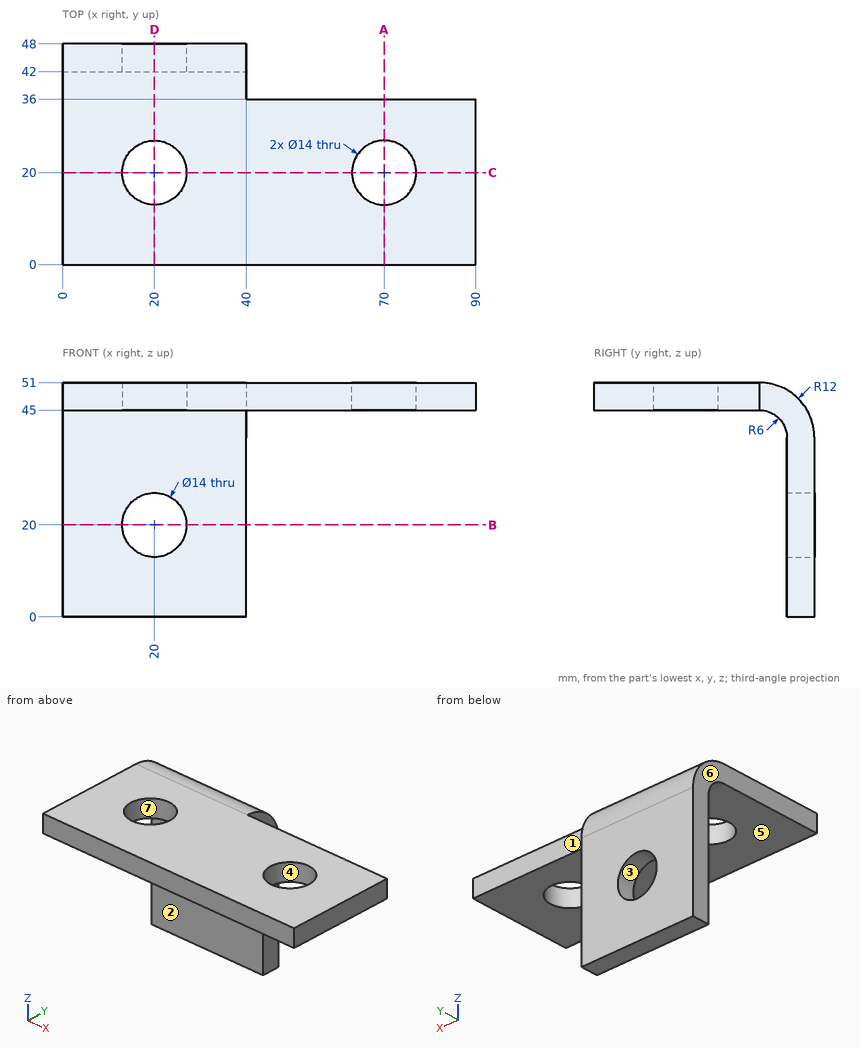
Drawing for the job (mm, zero at the part's lowest x, y, z). A direction names the side the tool comes from. Coordinates: 2 decimals unless noted, no trailing zeros. Order: outer loops, then holes, each group sorted by start corner. A loop starts at its lowest first (then second) coordinate and runs counter-clockwise, first axis right, second up. Notation, with made-up numbers: (-2.75, 26) -> (10.25, 26) arc R30 ccw to (10.25, 59) -> close; hole circle Ø5 at (51, 74.25). An arc over 180 degrees is marked (long way). Answer in a Markdown table with one row per item.
1) Drill centre lines: line 1 (X direction, y = 46.4, z = 20); line 2 (Y direction, x = 70, z = 47); line 3 (Z direction, x = 76.5, y = 23.5). Where is each one in solid material? Low to high.
Check values:
| item | result |
|---|---|
| line 1 | 0 to 13, 27 to 40 |
| line 2 | 0 to 13, 27 to 36 |
| line 3 | 45 to 51 |
2) Band-saw the part on C-C (y = 20). List the corners of the cut face in (x, z), and give its area (3 significant figures).
Check values:
| item | result |
|---|---|
| outline | (0, 45) -> (13, 45) -> (13, 51) -> (0, 51) -> close; (27, 45) -> (63, 45) -> (63, 51) -> (27, 51) -> close; (77, 45) -> (90, 45) -> (90, 51) -> (77, 51) -> close |
| area | 372 mm2 |
3) Band-saw the part on B-B (z = 20). List the corners of the cut face in (x, y), and give its area (3 significant figures).
Check values:
| item | result |
|---|---|
| outline | (0, 42) -> (13, 42) -> (13, 48) -> (0, 48) -> close; (27, 42) -> (40, 42) -> (40, 48) -> (27, 48) -> close |
| area | 156 mm2 |
4) Flat gauge pins, fed straight in: P1, Ø1.5, axis at x = 79.5, y = 24.5, coming from the -Z side; P2, Ø22.5, axis at x = 70, y = 20, coming from the +Z side; P3, Ø9.5, axis at y = 41.5, z = 23.5, coming from the +X side; P4, Ø19.5, axis at x = 28.5, z = 23.5, coming from the -Y side. Where does each tip first touch, or does it go through?
Check values:
| item | result |
|---|---|
| P1 | z = 45 |
| P2 | z = 51 |
| P3 | x = 40 |
| P4 | y = 42 |
5) Which spindle directions (+Z, -Z, +X, -X, +Y, -Y) get a long thin tool onto all of the face, cutting with end or side? Do the marked faces 1, 2 and 3. Say none if no direction does.
Check values:
| item | result |
|---|---|
| face 1 | +Z, -Z, +X, +Y |
| face 2 | -Z, +X, -X, -Y |
| face 3 | +Y, -Y |
6) Band-saw the part on D-D (x = 20). List the corners of the cut face in (y, z).
Check values:
| item | result |
|---|---|
| outline | (0, 45) -> (13, 45) -> (13, 51) -> (0, 51) -> close; (27, 45) -> (36, 45) arc R6 cw to (42, 39) -> (42, 27) -> (48, 27) -> (48, 39) arc R12 ccw to (36, 51) -> (27, 51) -> close; (42, 0) -> (48, 0) -> (48, 13) -> (42, 13) -> close |
7) Mould opens along X. For the marked faces 4, 5, 6 and 7 say: pulls with the +X half, pulls with the -X half, needs draft (parallel to the pull), parting line crosses it, or undercut.
Check values:
| item | result |
|---|---|
| face 4 | undercut |
| face 5 | needs draft |
| face 6 | pulls with the -X half |
| face 7 | undercut |
8) Band-saw the part on A-A (x = 70). List the corners of the cut face in (y, z), and give its area (3 significant figures).
Check values:
| item | result |
|---|---|
| outline | (0, 45) -> (13, 45) -> (13, 51) -> (0, 51) -> close; (27, 45) -> (36, 45) -> (36, 51) -> (27, 51) -> close |
| area | 132 mm2 |
